```python
from build123d import *

# Parameters (mm, degrees)
MODEL_R             = 38.5
MODEL_R_2           = 1.5
MODEL_R_3           = 1
MODEL_W             = 2
MODEL_H             = 8
MODEL_W_2           = 4
MODEL_H_2           = 11.4
BOSS_EXTRUDE1_DEPTH = 2


with BuildPart() as part:
    # Model → Boss-Extrude1 (new body)
    with BuildSketch(Plane.XY):
        with Locations((0, -0.073397172)):
            Circle(MODEL_R)
        with Locations((-23, 26.05)):
            Circle(MODEL_R_2, mode=Mode.SUBTRACT)
        with Locations((11.757144545, -32.719523315)):
            Circle(MODEL_R_2, mode=Mode.SUBTRACT)
        with Locations((11.757144545, 32.572728971)):
            Circle(MODEL_R_2, mode=Mode.SUBTRACT)
        with Locations((31.414701296, 12.426602828)):
            Circle(MODEL_R_3, mode=Mode.SUBTRACT)
        with Locations((31.414701296, -3.573397172)):
            Circle(MODEL_R_3, mode=Mode.SUBTRACT)
        with Locations((15.414701296, 12.426602828)):
            Circle(MODEL_R_3, mode=Mode.SUBTRACT)
        with Locations((15.414701296, -3.573397172)):
            Circle(MODEL_R_3, mode=Mode.SUBTRACT)
        with Locations((-23, -25.91)):
            Circle(MODEL_R_2, mode=Mode.SUBTRACT)
        with Locations((-15, -26.054159286)):
            Circle(MODEL_R_2, mode=Mode.SUBTRACT)
        with Locations((15, 25.907364941)):
            Circle(MODEL_R_2, mode=Mode.SUBTRACT)
        with Locations((-15, 25.907364941)):
            Circle(MODEL_R_2, mode=Mode.SUBTRACT)
        with Locations((15, -26.054159286)):
            Circle(MODEL_R_2, mode=Mode.SUBTRACT)
        with Locations((-12.5, -4.873397172)):
            Rectangle(MODEL_W, MODEL_H, mode=Mode.SUBTRACT)
        with Locations((-12.5, 18.626602828)):
            Rectangle(MODEL_W, MODEL_H, mode=Mode.SUBTRACT)
        with Locations((-6.5, -4.873397172)):
            Rectangle(MODEL_W_2, MODEL_H_2, mode=Mode.SUBTRACT)
        with Locations((6.5, -4.873397172)):
            Rectangle(MODEL_W_2, MODEL_H_2, mode=Mode.SUBTRACT)
        with BuildLine():
            Line((-2.25, 0), (-2.25, -9.746794345))
            ThreePointArc((-2.25, -9.746794345), (0, -11.996794345), (2.25, -9.746794345))
            Line((2.25, -9.746794345), (2.25, 0))
            ThreePointArc((2.25, 0), (0, 2.25), (-2.25, 0))
        make_face(mode=Mode.SUBTRACT)
    extrude(amount=BOSS_EXTRUDE1_DEPTH)


solid = part.part
```
Source: CAD feature listing. Evaluate the final solid. Frame: model axes, mm. Round coordinates to 2 decimals unless told otherwise and drop trailing zeros. Loops run counter-clockwise (first coordinate to the right, second up) from the corner with the lowest first, then second, coordinate; pieces in that order, holes last.
1. Ray query, L1, parallel to Y at x = -23, z = 1.5; L2, parallel to Y at x = 12, z = 0.15; L3, parallel to X at y = -26, z = 0.5. Return the intervals inside material, ascending.
2. Section query D-D on y = -14. Output: boundary loops of the cut face in (x, z).
3. Section query A-A on x = 0. Output: boundary loops of the cut face in (y, z).
4. Section query B-B on z = 1.4. Give the number of separate pieces and of enclosed holes in the cut face, and give its area (3 significant figures).
5. Mould query, pull axis Y, two halves, no side actions, for faces 1 (the cylindrical face through (11.43, 31.11, 0.99)), 2 (the cylindrical face through (36.722, 11.491, 0.986)), 3 (the cylindrical face through (-24.5, 26.1, 1)). Classes: released by +Y, released by -Y, zero draft, split by the parting line, or undercut.
6. Section query C-C on x = -23. Output: boundary loops of the cut face in (y, z).
7. Contact query for flat-ended pins moving along their axis: pin 1 (2.5 mm diameter, centred on x = -15, y = -26.05, fed in from -Z); pin 2 (0.6 mm diameter, centred on x = -12, z = 1, fed in from -Y); pin 3 (0.6 mm diameter, centred on y = -4, z = 1, fed in from +X); pin 4 (1 mm diameter, centred on y = -3.5, z = 1.5, fed in from -X). Output: stop coordinate, or through.
Answers below:
1. L1: y = -30.95 to -27.41, -24.41 to 24.55, 27.55 to 30.8
1. L2: y = -36.66 to -34.2, -31.24 to 31.09, 34.05 to 36.51
1. L3: x = -28.46 to -24.5, -21.5 to -16.5, -13.5 to 13.5, 16.5 to 28.46
2. outline: (-35.89, 0) - (35.89, 0) - (35.89, 2) - (-35.89, 2) - close
3. outline: (-38.57, 0) - (-12, 0) - (-12, 2) - (-38.57, 2) - close; (2.25, 0) - (38.43, 0) - (38.43, 2) - (2.25, 2) - close
4. separate pieces: 1
4. enclosed holes: 17
4. area: 4,400 mm2
5. face 1: undercut
5. face 2: split by the parting line
5. face 3: undercut
6. outline: (-30.95, 0) - (-27.41, 0) - (-27.41, 2) - (-30.95, 2) - close; (-24.41, 0) - (24.55, 0) - (24.55, 2) - (-24.41, 2) - close; (27.55, 0) - (30.8, 0) - (30.8, 2) - (27.55, 2) - close
7. pin 1: passes through
7. pin 2: stops at y = -36.75
7. pin 3: stops at x = 38.33
7. pin 4: stops at x = -38.39
